from build123d import *

# Parameters (mm, degrees)
SKETCH1_W                 = 21.7
SKETCH1_H                 = 33.6
BOSS_EXTRUDE1_DEPTH       = 3
SKETCH2_W                 = 18
SKETCH2_H                 = 3.5
CUT_EXTRUDE1_DEPTH        = 2
BOSS_EXTRUDE2_DEPTH       = 21.7
SKETCH4_W                 = 17.7
SKETCH4_H                 = 6.45
BOSS_EXTRUDE3_DEPTH       = 9.2
SKETCH5_W                 = 21.7
SKETCH5_H                 = 2
BOSS_EXTRUDE4_DEPTH       = 11
F_1_0MM_DOWEL_HOLE1_D     = 2.5
F_1_0MM_DOWEL_HOLE1_DEPTH = 9.248924226
F_1_0MM_DOWEL_HOLE1_TIP   = 0.751075774
CHAMFER1_SIZE             = 6.515477142
CHAMFER1_SIZE_2           = 0.8
CUT_EXTRUDE2_DEPTH        = 25.334389246
CUT_EXTRUDE2_DEPTH_BACK   = 1
SKETCH8_W                 = 21.7
SKETCH8_H                 = 35.6


with BuildPart() as part:
    # Sketch1 → Boss-Extrude1 (new body)
    with BuildSketch(Plane(origin=(0, 0, 0), x_dir=(1, 0, 0), z_dir=(0, 1, 0))):
        Rectangle(SKETCH1_W, SKETCH1_H)
    extrude(amount=BOSS_EXTRUDE1_DEPTH)

    # Sketch2 → Cut-Extrude1 (cut)
    with BuildSketch(Plane(origin=(0, 3, 0), x_dir=(1, 0, 0), z_dir=(0, 1, 0))):
        with Locations((0, -12.8)):
            Rectangle(SKETCH2_W, SKETCH2_H)
    extrude(amount=-CUT_EXTRUDE1_DEPTH, mode=Mode.SUBTRACT)

    # Sketch3 → Boss-Extrude2 (add)
    with BuildSketch(Plane(origin=(10.85, 0, 0), x_dir=(0, 0, -1), z_dir=(1, 0, 0))):
        Polygon((-8.8, 3), (16.8, 7.6), (16.8, 3), align=None)
    extrude(amount=-BOSS_EXTRUDE2_DEPTH)

    # Sketch4 → Boss-Extrude3 (add)
    with BuildSketch(Plane(origin=(0, 0, 0.27322177), x_dir=(1, 0, 0), z_dir=(0, 1, 0))):
        with Locations((0, 13.84822177)):
            Rectangle(SKETCH4_W, SKETCH4_H)
    extrude(amount=BOSS_EXTRUDE3_DEPTH)

    # Sketch5 → Boss-Extrude4 (add)
    with BuildSketch(Plane(origin=(0, 0, 0), x_dir=(1, 0, 0), z_dir=(0, 1, 0))):
        with Locations((0, -17.8)):
            Rectangle(SKETCH5_W, SKETCH5_H)
    extrude(amount=BOSS_EXTRUDE4_DEPTH)

    # Ø1.0mm Dowel Hole1
    with Locations(Plane.XY.offset(18.8)):
        with Locations((-8.35, 5.7), (8.35, 5.7)):
            Hole(F_1_0MM_DOWEL_HOLE1_D / 2, depth=F_1_0MM_DOWEL_HOLE1_DEPTH)
            with Locations((0, 0, -(F_1_0MM_DOWEL_HOLE1_DEPTH + F_1_0MM_DOWEL_HOLE1_TIP / 2))):  # 118° drill point
                Cone(0, F_1_0MM_DOWEL_HOLE1_D / 2, F_1_0MM_DOWEL_HOLE1_TIP, mode=Mode.SUBTRACT)

    # Chamfer1
    # the kernel refuses this chamfer: 6.515477142, 0.8 mm, written as the material it takes off along each edge
    with BuildSketch(Plane(origin=(25.785570178, 9.2, -10.35), x_dir=(0, 0.00468857506979086, -0.9999890085715017), z_dir=(-1, 0, 0))) as chamfer1_piece_1:
        Polygon((CHAMFER1_SIZE * 0.99998900863, CHAMFER1_SIZE * 0.00468857507006), (-CHAMFER1_SIZE_2 * 0.00468857506979, CHAMFER1_SIZE_2 * 0.999989008572), (0, 0), align=None)
    extrude(amount=51.571140357, mode=Mode.SUBTRACT)

    # Sketch8 → Cut-Extrude2 (cut, two sides: drawn at the far end of the back side and taken through both)
    with BuildSketch(Plane.XZ.offset(-CUT_EXTRUDE2_DEPTH_BACK)):
        with Locations((0, 1)):
            Rectangle(SKETCH8_W, SKETCH8_H)
    extrude(amount=CUT_EXTRUDE2_DEPTH + CUT_EXTRUDE2_DEPTH_BACK, mode=Mode.SUBTRACT)


solid = part.part
The listing builds one solid part. Answer for the finished solid, in the listing's coordinates (mm). A direction names the side the tool comes from. Round coordinates to 2 decimals unless told otherwise and drop trailing zeros. Write each loop counter-clockwise with the first axis right and the second up, starting at its lowest first coordinate (ties: lowest second). Pieces come first, ordered by that corner, then holes. Notation, with made-up numbers: (32, -0.75) - (89, -0.75) arc R12 cw to (89, 11.25) - close; hole circle Ø8 at (14, 84). An arc over 180 degrees is marked (long way). Use one line per item in the form item = value. Start each with the question number.
Item 1: A cutting plane is placed at A-A (x = 8.35). Write down the section's boundary in (y, z), plus the area to 3 significant figures.
Item 2: Find the intervals of material crossed by line 1 (Y direction, x = 8.35, z = 17.3); line 2 (Z direction, x = 5.75, y = 7.75); line 3 (Y direction, x = -6.5, z = 10), in increasing order. Write a range as [from, to].
Item 3: A tool of negligible diameter and unlimited length cuts with its end or side. For faces 5 (the flat face through (-8.85, 8, -14)), 6 (the cylindrical face through (-8.19, 6.94, 17.79)), 7 (the flat face through (0, 11, 18)), 8 (the flat face through (0, 3, 10)), 9 (the flat face through (9, 2, 13)), from which of +Z, -Z, +X, -X, +Y, -Y can it reach the whole face along a straight path? Write none if from no direction.
Item 4: Determine the mould class of faces 1 (the flat face through (0, 7, 16.8)), 2 (the flat face through (0, 2, 11.05)), 3 (the cylindrical face through (9.271, 6.545, 17.786)), 4 (the flat face through (0, 5, -16.8)) for opening direction Z: +Z half, -Z half, draft (parallel to the pull), parting line (faces both ways), or undercut.
Item 5: Flat-ended cylindrical pins translate along their axes: pin 1 Ø1 at (x, z) = (7, 14) entering from +Y; pin 2 Ø1.5 at (y, z) = (8.5, -12.5) entering from -X. Find the tip coordinate at first contact, or state that the pin passes through.
Item 6: A cutting plane is placed at B-B (z = 13.5). Write down the section's boundary in (x, y), plus the area to 3 significant figures.
Item 7: A cutting plane is placed at C-C (x = 0.5). Write down the section's boundary in (y, z), plus the area to 3 significant figures.
Item 8: A cutting plane is placed at D-D (y = 3.5). Write down the section's boundary in (x, z), plus the area to 3 significant figures.
The answers:
q1.outline = (1, -16.8) - (9.19, -16.8) - (8.4, -10.35) - (6.44, -10.35) - (3, 8.8) - (3, 11.05) - (1, 11.05) - close; (1, 14.55) - (3, 14.55) - (3, 16.8) - (4.45, 16.8) - (4.45, 18.8) - (1, 18.8) - close; (6.95, 16.8) - (11, 16.8) - (11, 18.8) - (6.95, 18.8) - close
q1.area = 146 mm^2
q2.line_1 = [1, 4.45], [6.95, 11]
q2.line_2 = [-16.8, -10.35], [16.8, 18.8]
q2.line_3 = [1, 3]
q3.face_5 = -X, +Y
q3.face_6 = +Z
q3.face_7 = +Z, -Z, +X, -X, +Y
q3.face_8 = +X, -X, +Y
q3.face_9 = +Y, -Y
q4.face_1 = undercut
q4.face_2 = undercut
q4.face_3 = draft
q4.face_4 = -Z half
q5.pin_1 = through
q5.pin_2 = -8.85
q6.outline = (-10.85, 1) - (-9, 1) - (-9, 3) - (-10.85, 3) - close; (9, 1) - (10.85, 1) - (10.85, 3) - (9, 3) - close
q6.area = 7.40 mm^2
q7.outline = (1, -16.8) - (9.19, -16.8) - (8.4, -10.35) - (6.44, -10.35) - (3, 8.8) - (3, 11.05) - (1, 11.05) - close; (1, 14.55) - (3, 14.55) - (3, 16.8) - (11, 16.8) - (11, 18.8) - (1, 18.8) - close
q7.area = 151 mm^2
q8.outline = (-10.85, -16.8) - (10.85, -16.8) - (10.85, 6.02) - (-10.85, 6.02) - close; (-10.85, 16.8) - (10.85, 16.8) - (10.85, 18.8) - (-10.85, 18.8) - close
q8.area = 539 mm^2
